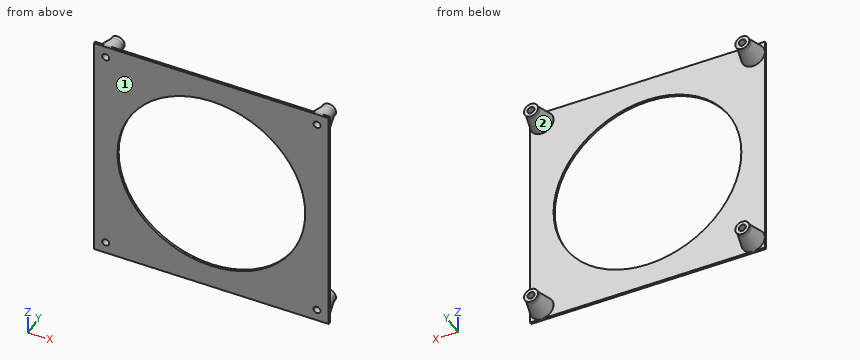
```python
from build123d import *

# Parameters (mm, degrees)
SKETCH1_W                 = 100
SKETCH1_H                 = 100
SKETCH1_R                 = 40
BOSS_EXTRUDE1_DEPTH       = 1
SKETCH2_R                 = 3
SKETCH2_R_2               = 1.5
BOSS_EXTRUDE2_DEPTH       = 9
CUT_EXTRUDE1_START        = 9
SKETCH2_3_R               = 1.5
CUT_EXTRUDE1_DEPTH        = 10
MIRROR2_COPY_1_SKETCH_R   = 3
MIRROR2_COPY_1_SKETCH_R_2 = 1.5
MIRROR2_COPY_1_DEPTH      = 9
MIRROR2_START             = 9
MIRROR2_COPY_2_SKETCH_R   = 1.5
MIRROR2_COPY_2_DEPTH      = 10
CHAMFER1_SIZE             = 2
CHAMFER1_SIZE_2           = 7.464101615


with BuildPart() as part:
    # Sketch1 → Boss-Extrude1 (new body)
    with BuildSketch(Plane(origin=(0, 0, 0), x_dir=(1, 0, 0), z_dir=(0, 1, 0))):
        Rectangle(SKETCH1_W, SKETCH1_H)
        with Locations(Location((0, 0, 0), (0, 0, 270))):
            Circle(SKETCH1_R, mode=Mode.SUBTRACT)
    extrude(amount=BOSS_EXTRUDE1_DEPTH)

    # Sketch2 → Boss-Extrude2 (add)
    # profile 1 of 2: a face of its own
    with BuildSketch(Plane(origin=(0, 1, 0), x_dir=(1, 0, 0), z_dir=(0, 1, 0))):
        with Locations(Location((-45, -45, 0), (0, 0, 270))):
            Circle(SKETCH2_R)
        with Locations((-45, -45)):
            Circle(SKETCH2_R_2, mode=Mode.SUBTRACT)
    # profile 2 of 2: a face of its own
    with BuildSketch(Plane(origin=(0, 1, 0), x_dir=(1, 0, 0), z_dir=(0, 1, 0))):
        with Locations((-45, -45)):
            Circle(SKETCH2_R_2)
    boss_extrude2 = extrude(amount=BOSS_EXTRUDE2_DEPTH)

    # Sketch2<3> → Cut-Extrude1 (cut)
    with BuildSketch(Plane(origin=(0, 1, 0), x_dir=(1, 0, 0), z_dir=(0, 1, 0)).offset(CUT_EXTRUDE1_START)):
        with Locations(Location((-45, -45, 0), (0, 0, 270))):
            Circle(SKETCH2_3_R)
    cut_extrude1 = extrude(amount=-CUT_EXTRUDE1_DEPTH, mode=Mode.SUBTRACT)

    # Mirror1: Boss-Extrude2, Cut-Extrude1 across plane
    add(boss_extrude2.mirror(Plane(origin=(0, 0, 0), x_dir=(0, 0, 1), z_dir=(1, 0, 0))))
    add(cut_extrude1.mirror(Plane(origin=(0, 0, 0), x_dir=(0, 0, 1), z_dir=(1, 0, 0))), mode=Mode.SUBTRACT)

    # Mirror2: Boss-Extrude2, Cut-Extrude1 across plane
    add(boss_extrude2.mirror(Plane.XY))
    add(cut_extrude1.mirror(Plane.XY), mode=Mode.SUBTRACT)

    # Mirror2 copy 1 sketch → Mirror2 copy 1 (add)
    # profile 1 of 2: a face of its own
    with BuildSketch(Plane(origin=(0, 1, 0), x_dir=(-1, 0, 0), z_dir=(0, 1, 0))):
        with Locations(Location((-45, -45, 0), (0, 0, 270))):
            Circle(MIRROR2_COPY_1_SKETCH_R)
        with Locations((-45, -45)):
            Circle(MIRROR2_COPY_1_SKETCH_R_2, mode=Mode.SUBTRACT)
    # profile 2 of 2: a face of its own
    with BuildSketch(Plane(origin=(0, 1, 0), x_dir=(-1, 0, 0), z_dir=(0, 1, 0))):
        with Locations((-45, -45)):
            Circle(MIRROR2_COPY_1_SKETCH_R_2)
    extrude(amount=MIRROR2_COPY_1_DEPTH)

    # Mirror2 copy 2 sketch → Mirror2 copy 2 (cut)
    with BuildSketch(Plane(origin=(0, 1, 0), x_dir=(-1, 0, 0), z_dir=(0, 1, 0)).offset(MIRROR2_START)):
        with Locations(Location((-45, -45, 0), (0, 0, 270))):
            Circle(MIRROR2_COPY_2_SKETCH_R)
    extrude(amount=-MIRROR2_COPY_2_DEPTH, mode=Mode.SUBTRACT)

    # Chamfer1
    # the kernel refuses this chamfer: 7.464101615, 2 mm, written as the material it adds along each edge
    with BuildSketch(Plane(origin=(-45, 1, 45), x_dir=(0, 0, 1), z_dir=(-1, 0, 0))) as chamfer1_piece_1_section:
        Polygon((3 + CHAMFER1_SIZE, 0), (3, CHAMFER1_SIZE_2), (3, 0), align=None)
    chamfer1_piece_1 = revolve(axis=Axis((-45, 1, 45), (0, 1, 0)), mode=Mode.PRIVATE)
    chamfer1_piece_1 = split(chamfer1_piece_1, bisect_by=Plane(origin=(-45, 4.716774414, 50), z_dir=(0, 0, -1)), keep=Keep.TOP, mode=Mode.PRIVATE)
    chamfer1_piece_1 = split(chamfer1_piece_1, bisect_by=Plane(origin=(-50, 4.716774414, 41.057012278), z_dir=(1, 0, 0)), keep=Keep.TOP, mode=Mode.PRIVATE)
    add(chamfer1_piece_1)
    with BuildSketch(Plane(origin=(45, 1, 45), x_dir=(0, 0, 1), z_dir=(1, 0, 0))) as chamfer1_piece_2_section:
        Polygon((3 + CHAMFER1_SIZE, 0), (3, -CHAMFER1_SIZE_2), (3, 0), align=None)
    chamfer1_piece_2 = revolve(axis=Axis((45, 1, 45), (0, -1, 0)), mode=Mode.PRIVATE)
    chamfer1_piece_2 = split(chamfer1_piece_2, bisect_by=Plane(origin=(45, 4.716774414, 50), z_dir=(0, 0, -1)), keep=Keep.TOP, mode=Mode.PRIVATE)
    chamfer1_piece_2 = split(chamfer1_piece_2, bisect_by=Plane(origin=(50, 4.716774414, 41.057012278), z_dir=(-1, 0, 0)), keep=Keep.TOP, mode=Mode.PRIVATE)
    add(chamfer1_piece_2)
    with BuildSketch(Plane(origin=(45, 1, -45), x_dir=(0, 0, -1), z_dir=(1, 0, 0))) as chamfer1_piece_3_section:
        Polygon((3 + CHAMFER1_SIZE, 0), (3, CHAMFER1_SIZE_2), (3, 0), align=None)
    chamfer1_piece_3 = revolve(axis=Axis((45, 1, -45), (0, 1, 0)), mode=Mode.PRIVATE)
    chamfer1_piece_3 = split(chamfer1_piece_3, bisect_by=Plane(origin=(50, 4.716774414, -41.057012278), z_dir=(-1, 0, 0)), keep=Keep.TOP, mode=Mode.PRIVATE)
    chamfer1_piece_3 = split(chamfer1_piece_3, bisect_by=Plane(origin=(45, 4.716774414, -50), z_dir=(0, 0, 1)), keep=Keep.TOP, mode=Mode.PRIVATE)
    add(chamfer1_piece_3)
    with BuildSketch(Plane(origin=(-45, 1, -45), x_dir=(0, 0, -1), z_dir=(-1, 0, 0))) as chamfer1_piece_4_section:
        Polygon((3 + CHAMFER1_SIZE, 0), (3, -CHAMFER1_SIZE_2), (3, 0), align=None)
    chamfer1_piece_4 = revolve(axis=Axis((-45, 1, -45), (0, -1, 0)), mode=Mode.PRIVATE)
    chamfer1_piece_4 = split(chamfer1_piece_4, bisect_by=Plane(origin=(-50, 4.716774414, -41.057012278), z_dir=(1, 0, 0)), keep=Keep.TOP, mode=Mode.PRIVATE)
    chamfer1_piece_4 = split(chamfer1_piece_4, bisect_by=Plane(origin=(-45, 4.716774414, -50), z_dir=(0, 0, 1)), keep=Keep.TOP, mode=Mode.PRIVATE)
    add(chamfer1_piece_4)


solid = part.part
```
Build history of the part. All positions in model axes, mm. Face numbers are marked on the shaded views. Round coordinates to 2 decimals unless told otherwise and drop trailing zeros. Loops run counter-clockwise (first coordinate to the right, second up) from the corner with the lowest first, then second, coordinate; pieces in that order, holes last. Notation, with made-up numbers: M 76,63 L 111,63 A34 cw 111,101 Z; hole C 18.5,-21 d8. An arc over 180 degrees is marked long. Answer as CSV lines item,"result".
1. Cut at B-B on z = 0. Write the cut outline in (x, y), then the cut area to 3 significant figures.
Resolved:
outline,"M -50,0 L -40,0 L -40,1 L -50,1 Z; M 40,0 L 50,0 L 50,1 L 40,1 Z"
area,"20.0 mm²"
2. Cut at C-C on y = 4.25. Write the cut outline in (x, z).
Resolved:
outline,"C -45,-45 d8.26; C -45,45 d8.26; C 45,-45 d8.26; C 45,45 d8.26; hole C -45,-45 d3; hole C -45,45 d3; hole C 45,-45 d3; hole C 45,45 d3"
3. Cut at A-A on x = 0. Write the cut outline in (y, z), then the cut area to 3 significant figures.
Resolved:
outline,"M 0,-50 L 1,-50 L 1,-40 L 0,-40 Z; M 0,40 L 1,40 L 1,50 L 0,50 Z"
area,"20.0 mm²"
4. Flat gauge pins, fed straight in: P1, Ø10, axis at x = -3, z = 39, coming from the +Y side; P2, Ø2.5, axis at x = -45, z = 45, coming from the -Y side. Where does each tip first touch, or does it go through?
Resolved:
P1,"stops at y = 1"
P2,"passes through"
5. Wall check: probe 1 along X at (y, z) = (6, -45); probe 2 along Z at (x, y) = (44.5, 6); probe 3 along X at (y, z) = (6.75, 45). Give the ranges that are in metal, low to high. Write a range as [from, to].
Resolved:
probe 1,"x = [-48.66, -46.5], [-43.5, -41.34], [41.34, 43.5], [46.5, 48.66]"
probe 2,"z = [-48.63, -46.41], [-43.59, -41.37], [41.37, 43.59], [46.41, 48.63]"
probe 3,"x = [-48.46, -46.5], [-43.5, -41.54], [41.54, 43.5], [46.5, 48.46]"
6. Two-plate mould, pull along X, no slides. Class the marked faces 1 and 2: released by +X, released by -X, zero draft, split by the parting line, or undercut.
Resolved:
face 1,"zero draft"
face 2,"undercut"
